from build123d import *

# Parameters (mm, degrees)
SKETCH1_W           = 6
SKETCH1_H           = 6
BOSS_EXTRUDE1_DEPTH = 20


with BuildPart() as part:
    # Sketch1 → Boss-Extrude1 (new body)
    with BuildSketch(Plane(origin=(0, 0, 0), x_dir=(1, 0, 0), z_dir=(0, 1, 0))):
        Rectangle(SKETCH1_W, SKETCH1_H)
    extrude(amount=BOSS_EXTRUDE1_DEPTH)

    # Sketch3 → Cut-Revolve1 (revolve, cut)
    with BuildSketch(Plane(origin=(0, 20, 0), x_dir=(1, 0, 0), z_dir=(0, 1, 0))):
        with BuildLine():
            Line((-2, 0), (2, 0))
            ThreePointArc((2, 0), (0, 2), (-2, 0))
        make_face()
    revolve(axis=Axis((-2, 20, 0), (1, 0, 0)), mode=Mode.SUBTRACT)


solid = part.part
Verification items for the finished model (mm, model axes). Coordinates: 2 decimals unless noted, no trailing zeros. Order: outer loops, then holes, each group sorted by start corner. A loop starts at its lowest first (then second) coordinate and runs counter-clockwise, first axis right, second up. Notation, with made-up numbers: (-24, -37.5) -> (14, -37.5) arc R16 ccw to (14, -8.5) -> close; hole circle Ø8 at (-2.5, 60.5). An arc over 180 degrees is marked (long way). Use CSV: the item, a comma, the result in double quotes. Start each with the question number.
Q1. Thickness scan on line 1 along Z through (x, y) = (-0.85, 18.5); line 2 along Y through (x, z) = (-0.95, 1.05); line 3 along Y through (x, z) = (0.8, 0.5). Record the ranges inside material, lowest first.
Q2. Section check A-A, the plane z = 1.15. Record the cut outline in (x, y), and give its area (3 significant figures).
Q3. Section check B-B, the plane x = 1.5. Record the cut outline in (y, z).
Returned:
1,line 1,"z = -3 to -1.01, 1.01 to 3"
1,line 2,"y = 0 to 18.59"
1,line 3,"y = 0 to 18.24"
2,outline,"(-3, 0) -> (3, 0) -> (3, 20) -> (1.64, 20) arc R1.64 cw to (-1.64, 20) -> (-3, 20) -> close"
2,area,"116 mm^2"
3,outline,"(0, -3) -> (20, -3) -> (20, -1.32) arc R1.32 cw to (20, 1.32) -> (20, 3) -> (0, 3) -> close"
